Verification items for the finished model (mm, model axes). A direction names the side the tool comes from. Give positions to 0.01 mm unless a question says otherwise; leave off trailing zeros. Write each loop counter-clockwise with the first axis right and the second up, starting at its lowest first coordinate (ties: lowest second). Pieces come first, ordered by that corner, then holes. Notation, with made-up numbers: (79.5, -28) - (122.5, -28) arc R28 ccw to (122.5, -1) - close; hole circle Ø5 at (-34, 78). An arc over 180 degrees is marked (long way). Answer as a JSON object with one key per item and string values. Group by question number.
Item 1: Sectioned sample at A-A, the plane x = -51. Record the boundary of the cut face in (y, z), and give its area (3 significant figures).
Item 2: Sectioned sample at B-B, the plane z = 17.5. Record the boundary of the cut face in (x, y).
Item 3: Sectioned sample at D-D, the plane x = 1. Record the boundary of the cut face in (y, z), and give its area (3 significant figures).
Item 4: Draft check along X on faces 1 (the face through (30, 30, -1)), 2 (the face through (40, 14, 12)), 3 (the face through (-9.39, 33.04, -1.57)), 4 (the face through (-51, 30, 15)). Enter one of: +X half, -X half, draft (parallel to the pull), parting line (faces both ways), or undercut.
Item 5: Sectioned sample at C-C, the plane y = 9. Record the boundary of the cut face in (x, z).
Item 6: Tool access check on faces 5 (the face through (32, 18, -12)), 6 (the face through (-51, 33, 10)), 7 (the face through (30.323, 14.79, 7.493)), 8 (the face through (-20, 15, 5)). Record the directions out of +Z, -Z, +X, -X, +Y, -Y that give a thin tool (end or side, any length) a straight path to the whole face; none if there is none.
Item 7: Scan lines: line 1 along X through (y, z) = (21.5, 0); line 2 along X through (y, z) = (18.5, -3.5); line 3 along Z through (x, y) = (-51, 32.8). Record each from-to range of solid material in increasing order. Write a range as [from, to].
Item 8: Go/stop test with flat-tipped pins: pin 1 (6 mm diameter, centred on x = -1.5, z = 6.5, fed in from -Y); pin 2 (20 mm diameter, centred on y = 10, z = 11.5, fed in from +X); pin 3 (1.2 mm diameter, centred on y = 17.5, z = -12.5, fed in from -X); pin 4 (5 mm diameter, centred on x = 39.5, z = -10, fed in from +Y). Record where each tip stops, or that it passes through.
```python
from build123d import *

# Parameters (mm, degrees)
SALIENTE_EXTRUIR1_DEPTH    = 30
SALIENTE_EXTRUIR2_START    = -30
SALIENTE_EXTRUIR2_DEPTH    = 30
CORTAR_EXTRUIR2_DEPTH      = 56.901699437
CORTAR_EXTRUIR2_DEPTH_BACK = 56.901699437
CORTAR_EXTRUIR3_START      = -30
CORTAR_EXTRUIR3_DEPTH      = 30
SALIENTE_EXTRUIR3_DEPTH    = 6
CROQUIS13_R                = 1.5
CORTAR_EXTRUIR6_DEPTH      = 75.303431953
REDONDEO3_R                = 3
REDONDEO4_R                = 3


with BuildPart() as part:
    # Croquis1 → Saliente-Extruir1 (new body)
    with BuildSketch(Plane(origin=(0, 0, 0), x_dir=(1, 0, 0), z_dir=(0, 1, 0))):
        with BuildLine():
            Line((40, -25), (40, 0))
            ThreePointArc((40, 0), (32.043096437, 9.789063129), (20.83484861, 4))
            Line((20.83484861, 4), (11.313708499, 4))
            ThreePointArc((11.313708499, 4), (0, 12), (-11.313708499, 4))
            Line((-11.313708499, 4), (-20.83484861, 4))
            ThreePointArc((-20.83484861, 4), (-32.043096437, 9.789063129), (-40, 0))
            Line((-40, 0), (-40, -25))
            Line((-40, -25), (40, -25))
        make_face()
    extrude(amount=SALIENTE_EXTRUIR1_DEPTH)

    # Croquis3 → Saliente-Extruir2 (add)
    with BuildSketch(Plane(origin=(0, 30, 0), x_dir=(1, 0, 0), z_dir=(0, 1, 0)).offset(SALIENTE_EXTRUIR2_START)):
        with BuildLine():
            Line((-32, 9.797958971), (-32, 13.797958971))
            Line((-32, 13.797958971), (-28, 13.797958971))
            Line((-28, 13.797958971), (-28, 9.797958971))
            ThreePointArc((-28, 9.797958971), (-30, 10), (-32, 9.797958971))
        make_face()
        with BuildLine():
            Line((28, 9.797958971), (28, 13.797958971))
            Line((28, 13.797958971), (32, 13.797958971))
            Line((32, 13.797958971), (32, 9.797958971))
            ThreePointArc((32, 9.797958971), (30, 10), (28, 9.797958971))
        make_face()
    extrude(amount=SALIENTE_EXTRUIR2_DEPTH)

    # Croquis4 → Cortar-Extruir2 (cut, two sides: drawn at the far end of the back side and taken through both)
    with BuildSketch(Plane(origin=(0, 30, 0), x_dir=(1, 0, 0), z_dir=(0, 1, 0)).offset(-CORTAR_EXTRUIR2_DEPTH_BACK)):
        with BuildLine():
            Line((-30.5, 7.483314774), (-30.5, 14.654769407))
            Line((-30.5, 14.654769407), (-29.5, 14.654769407))
            Line((-29.5, 14.654769407), (-29.5, 7.483314774))
            ThreePointArc((-29.5, 7.483314774), (-30, -7.5), (-30.5, 7.483314774))
        make_face()
        with BuildLine():
            Line((29.5, 7.483314774), (29.5, 14.654769407))
            Line((29.5, 14.654769407), (30.5, 14.654769407))
            Line((30.5, 14.654769407), (30.5, 7.483314774))
            ThreePointArc((30.5, 7.483314774), (30, -7.5), (29.5, 7.483314774))
        make_face()
    extrude(amount=CORTAR_EXTRUIR2_DEPTH + CORTAR_EXTRUIR2_DEPTH_BACK, mode=Mode.SUBTRACT)

    # Croquis5 → Cortar-Extruir3 (cut)
    with BuildSketch(Plane(origin=(0, 30, 0), x_dir=(1, 0, 0), z_dir=(0, 1, 0)).offset(CORTAR_EXTRUIR3_START)):
        with BuildLine():
            Line((-20, 0), (-20, -10))
            Line((-20, -10), (20, -10))
            Line((20, -10), (20, 0))
            ThreePointArc((20, 0), (20.210936871, 2.043096437), (20.83484861, 4))
            Line((20.83484861, 4), (20.83484861, 13.99599321))
            Line((20.83484861, 13.99599321), (-20.83484861, 13.99599321))
            Line((-20.83484861, 13.99599321), (-20.83484861, 4))
            ThreePointArc((-20.83484861, 4), (-20.210936871, 2.043096437), (-20, 0))
        make_face()
    extrude(amount=CORTAR_EXTRUIR3_DEPTH, mode=Mode.SUBTRACT)

    # Croquis12 → Saliente-Extruir3 (add)
    with BuildSketch(Plane(origin=(0, 30, 0), x_dir=(1, 0, 0), z_dir=(0, 1, 0))):
        with BuildLine():
            Line((40, -25), (-40, -25))
            Line((-40, -25), (-57, -25))
            ThreePointArc((-57, -25), (-59.121320344, -24.121320344), (-60, -22))
            Line((-60, -22), (-60, -13))
            ThreePointArc((-60, -13), (-59.121320344, -10.878679656), (-57, -10))
            Line((-57, -10), (-45, -10))
            ThreePointArc((-45, -10), (-41.464466094, -8.535533906), (-40, -5))
            Line((-40, -5), (-40, 0))
            ThreePointArc((-40, 0), (-37.745966692, 6.32455532), (-32, 9.797958971))
            Line((-32, 9.797958971), (-32, 13.797958971))
            Line((-32, 13.797958971), (32, 13.797958971))
            Line((32, 13.797958971), (32, 9.797958971))
            ThreePointArc((32, 9.797958971), (37.745966692, 6.32455532), (40, 0))
            Line((40, 0), (40, -5))
            ThreePointArc((40, -5), (41.464466094, -8.535533906), (45, -10))
            Line((45, -10), (57, -10))
            ThreePointArc((57, -10), (59.121320344, -10.878679656), (60, -13))
            Line((60, -13), (60, -22))
            ThreePointArc((60, -22), (59.121320344, -24.121320344), (57, -25))
            Line((57, -25), (40, -25))
        make_face()
    extrude(amount=SALIENTE_EXTRUIR3_DEPTH)

    # Croquis13 → Cortar-Extruir6 (cut, through all)
    with BuildSketch(Plane(origin=(0, 36, 0), x_dir=(1, 0, 0), z_dir=(0, 1, 0))):
        with Locations(Location((51, -17.5, 0), (0, 0, 270))):
            Circle(CROQUIS13_R)
        with Locations(Location((-51, -17.5, 0), (0, 0, 90))):
            Circle(CROQUIS13_R)
        with Locations(Location((-10.655547213, 2.375143361, 0), (0, 0, 270))):
            Circle(CROQUIS13_R)
        with Locations(Location((10.655547213, 2.375143361, 0), (0, 0, 90))):
            Circle(CROQUIS13_R)
    extrude(amount=-CORTAR_EXTRUIR6_DEPTH, mode=Mode.SUBTRACT)

    # Redondeo3
    redondeo3_edges = [part.edges().sort_by_distance(p)[0] for p in [
        (40, 30, 15),
    ]]
    fillet(redondeo3_edges, radius=REDONDEO3_R)

    # Redondeo4
    redondeo4_edges = [part.edges().sort_by_distance(p)[0] for p in [
        (-40, 30, 15),
    ]]
    fillet(redondeo4_edges, radius=REDONDEO4_R)


solid = part.part
```
Geometry check:
{
 "1": {"outline": "(30, 10) - (36, 10) - (36, 16) - (30, 16) - close; (30, 19) - (36, 19) - (36, 25) - (30, 25) - close", "area": "72.0 mm^2"},
 "2": {"outline": "(-60, 30) - (-52.5, 30) - (-52.5, 36) - (-60, 36) - close; (-49.5, 30) - (-43, 30) arc R3 cw to (-40, 27) - (-40, 0) - (40, 0) - (40, 27) arc R3 cw to (43, 30) - (49.5, 30) - (49.5, 36) - (-49.5, 36) - close; (52.5, 30) - (60, 30) - (60, 36) - (52.5, 36) - close"},
 "3": {"outline": "(0, 10) - (30, 10) - (30, -13.8) - (36, -13.8) - (36, 25) - (0, 25) - close", "area": "683 mm^2"},
 "4": {"face 1": "undercut", "face 2": "+X half", "face 3": "undercut", "face 4": "draft"},
 "5": {"outline": "(-40, 0) arc R10 ccw to (-32, -9.8) - (-32, -13.8) - (-30.5, -13.8) - (-30.5, -7.48) arc R7.5 cw (long way) to (-29.5, -7.48) - (-29.5, -13.8) - (-28, -13.8) - (-28, -9.8) arc R10 ccw to (-20, 0) - (-20, 10) - (20, 10) - (20, 0) arc R10 ccw to (28, -9.8) - (28, -13.8) - (29.5, -13.8) - (29.5, -7.48) arc R7.5 cw (long way) to (30.5, -7.48) - (30.5, -13.8) - (32, -13.8) - (32, -9.8) arc R10 ccw to (40, 0) - (40, 25) - (-40, 25) - close"},
 "6": {"face 5": "-Z, +X, +Y, -Y", "face 6": "-Z, -X, +Y, -Y", "face 7": "-Y", "face 8": "-Z, -Y"},
 "7": {"line 1": "[-40, -37.5], [-22.5, -20], [20, 22.5], [37.5, 40]", "line 2": "[-39.37, -36.63], [-23.37, -20.63], [20.63, 23.37], [36.63, 39.37]", "line 3": "[10, 16], [19, 25]"},
 "8": {"pin 1": "y = 30", "pin 2": "x = 40", "pin 3": "x = -32", "pin 4": "through"}
}
